```python
from build123d import *

# Parameters (mm, degrees)
F1_DEPTH = 5


with BuildPart() as f1:
    # F0 (on Top) → F1 (new body)
    with BuildSketch(Plane.XY):
        with BuildLine():
            ThreePointArc((-7.0000001151, -12.688577613), (-3.2259131968, -9.2935934897), (-0.8003333333, -4.8341976124))
            ThreePointArc((-0.8003333333, -4.8341976124), (-1.9050962629, -4.5144887007), (-2.9049071205, -3.9460758509))
            ThreePointArc((-2.9049071205, -3.9460758509), (-12.814429581, -8.8589229177), (-23.6491115752, -6.635329479))
            Line((-23.6491115752, -6.635329479), (-27.1270159685, -8.8281075945))
            ThreePointArc((-27.1270159685, -8.8281075945), (-17.8255747432, -14.7314672511), (-7.0000001151, -12.688577613))
        make_face()
        with BuildLine():
            ThreePointArc((-0.8003333333, -4.8341976124), (-0.3863117112, -3.382323846), (-0.1203333333, -1.8961856156))
            ThreePointArc((-0.1203333333, -1.8961856156), (-0.5698724421, -1.8125245929), (-0.9864055845, -1.623885471))
            ThreePointArc((-0.9864055845, -1.623885471), (-1.8941223069, -2.8275560443), (-2.9049071205, -3.9460758509))
            ThreePointArc((-2.9049071205, -3.9460758509), (-1.9050962629, -4.5144887007), (-0.8003333333, -4.8341976124))
        make_face()
        with BuildLine():
            ThreePointArc((0.9864055845, 1.623885471), (1.6559243054, 0.9316193937), (1.9, 0))
            ThreePointArc((1.9, 0), (1.300262794, -1.3853940474), (-0.1203333333, -1.8961856156))
            ThreePointArc((-0.1203333333, -1.8961856156), (-0.3863117112, -3.382323846), (-0.8003333333, -4.8341976124))
            ThreePointArc((-0.8003333333, -4.8341976124), (3.1692559589, -3.737086655), (4.9, 0))
            ThreePointArc((4.9, 0), (4.3728734769, 2.2108771008), (2.9049071205, 3.9460758509))
            ThreePointArc((2.9049071205, 3.9460758509), (1.8941223069, 2.8275560443), (0.9864055845, 1.623885471))
        make_face()
        with BuildLine():
            ThreePointArc((-0.9864055845, -1.623885471), (-1.8125245929, 0.5698724421), (0.1203333333, 1.8961856156))
            ThreePointArc((0.1203333333, 1.8961856156), (0.3863117112, 3.382323846), (0.8003333333, 4.8341976124))
            ThreePointArc((0.8003333333, 4.8341976124), (-4.5144887007, 1.9050962629), (-2.9049071205, -3.9460758509))
            ThreePointArc((-2.9049071205, -3.9460758509), (-1.8941223069, -2.8275560443), (-0.9864055845, -1.623885471))
        make_face()
        with BuildLine():
            ThreePointArc((0.1203333333, 1.8961856156), (0.5698724421, 1.8125245929), (0.9864055845, 1.623885471))
            ThreePointArc((0.9864055845, 1.623885471), (1.8941223069, 2.8275560443), (2.9049071205, 3.9460758509))
            ThreePointArc((2.9049071205, 3.9460758509), (1.9050962629, 4.5144887007), (0.8003333333, 4.8341976124))
            ThreePointArc((0.8003333333, 4.8341976124), (0.3863117112, 3.382323846), (0.1203333333, 1.8961856156))
        make_face()
        with BuildLine():
            ThreePointArc((0.8003333333, 4.8341976124), (1.9050962629, 4.5144887007), (2.9049071205, 3.9460758509))
            ThreePointArc((2.9049071205, 3.9460758509), (12.814429581, 8.8589229177), (23.6491115752, 6.635329479))
            Line((23.6491115752, 6.635329479), (27.1270159685, 8.8281075945))
            ThreePointArc((27.1270159685, 8.8281075945), (17.8255747198, 14.7314672556), (7.0000000748, 12.6885775876))
            ThreePointArc((7.0000000748, 12.6885775876), (3.225913182, 9.2935934709), (0.8003333333, 4.8341976124))
        make_face()
    extrude(amount=F1_DEPTH)


solid = f1.part
```
Model file for the job. Use its own axes, mm. Give positions to 0.01 mm unless a question says otherwise; leave off trailing zeros. Loops run counter-clockwise (first coordinate to the right, second up) from the corner with the lowest first, then second, coordinate; pieces in that order, holes last. Notation, with made-up numbers: M 16.5,-22.75 L 28.5,-22.75 A14 cw 28.5,-0.75 Z; hole C 81.25,11.5 d7. An arc over 180 degrees is marked long. Use one line per item in the form item = value.
Item 1: Drill centre lines: L1, parallel to Y at x = 0, z = 2.1; L2, parallel to X at y = -1.25, z = 4.3; L3, parallel to Y at x = 15, z = 2.55. Where is each one in solid material? Low to high.
Filled in:
L1 = -4.9 to -1.9, 1.9 to 4.9
L2 = -4.74 to -1.43, 1.43 to 4.74
L3 = 9 to 15
Item 2: Slice it at A-A on z = 3.2. List the corners of the cut face in (x, y), and give its area (3 significant figures).
Filled in:
outline = M -27.13,-8.83 A15 ccw -0.8,-4.83 A4.9 ccw 2.9,3.95 A17 cw 23.65,6.64 L 27.13,8.83 A15 ccw 0.8,4.83 A4.9 ccw -2.9,-3.95 A17 cw -23.65,-6.64 Z; hole C 0,0 d3.8
area = 336 mm^2
Item 3: Slice it at B-B on y = -0.75. List the corners of the cut face in (x, z), and give its area (3 significant figures).
Filled in:
outline = M -4.84,0 L -1.75,0 L -1.75,5 L -4.84,5 Z; M 1.75,0 L 4.84,0 L 4.84,5 L 1.75,5 Z
area = 31.0 mm^2
Item 4: Slice it at C-C on x = -23. List the corners of the cut face in (y, z), and give its area (3 significant figures).
Filled in:
outline = M -12.69,0 L -7,0 L -7,5 L -12.69,5 Z
area = 28.4 mm^2
Item 5: Two-plate mould, pull along X, no slides. Class faces 1 (the flat face through (-25.364, -7.716, 2.465)), 2 (the cylindrical face through (-12.66, -8.84, 2.46)), 3 (the flat face through (-2.1, 0.1, 0)): released by +X, released by -X, zero draft, split by the parting line, or undercut.
Filled in:
face_1 = released by -X
face_2 = undercut
face_3 = zero draft
Item 6: Flat gauge pins, fed straight in: pin 1 Ø1.5 at (x, z) = (17, 3.5) entering from -Y; pin 2 Ø1 at (x, z) = (-13.5, 4) entering from -Y; pin 3 Ø1 at (y, z) = (0, 1.5) entering from +X. Where does each tip first touch, or does it go through?
Filled in:
pin_1 = 8.78
pin_2 = -14.97
pin_3 = 4.9
Item 7: Slice it at D-D on y = -10.5. List the corners of the cut face in (x, z).
Filled in:
outline = M -25.71,0 L -4.29,0 L -4.29,5 L -25.71,5 Z
